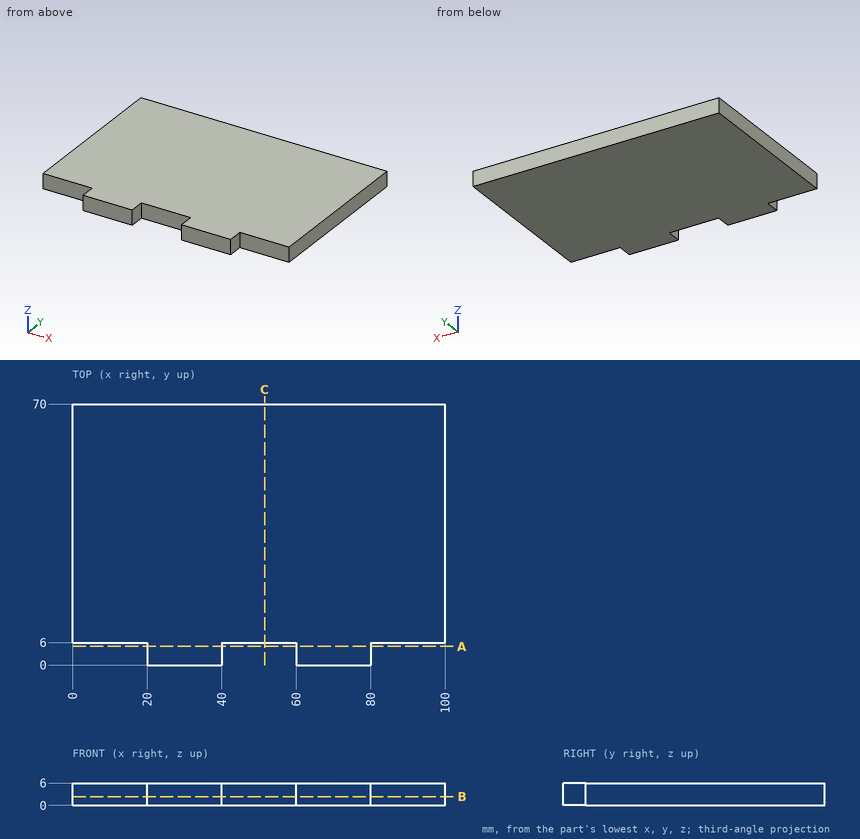
Input: dimensioned drawing with shaded views. Units: mm. Origin: part minimum x, y, z. Give positions to 0.01 mm unless a question says otherwise; leave off trailing zeros. Write each loop counter-clockwise with the first axis right and the second up, starting at its lowest first coordinate (ties: lowest second). Pieces come first, ordered by that corner, then holes. Notation, with made-up numbers: M 57.5,49.25 L 100.5,49.25 A20 ccw 100.5,57.25 Z; hole C 60.5,70 d9. An arc over 180 degrees is marked long. Return JSON: item names as keys, results as strings. Group by question number.
1) Material intervals for line 1 along Y through (x, z) = (15, 1.25), sorted ascending. Write a range as [from, to].
2) Pin query (flat end, axial travel): P1, Ø1.8, axis at y = 2.5, z = 2, coming from the +X side; P2, Ø2, axis at x = 69.5, y = 62, coming from the -Z side. Return the tip coordinate at first contact, or that it passes through.
3) Cut plane B-B, the plane z = 2.35. Output: boundary loops of the cut face in (x, y).
4) Cut plane C-C, the plane x = 51.5. Output: boundary loops of the cut face in (y, z), plus the area to 3 significant figures.
5) Cut plane A-A, the plane y = 5. Output: boundary loops of the cut face in (x, z).
Recorded:
{
 "1": {"line 1": "y = [6, 70]"},
 "2": {"P1": "stops at x = 80", "P2": "stops at z = 0"},
 "3": {"outline": "M 0,6 L 20,6 L 20,0 L 40,0 L 40,6 L 60,6 L 60,0 L 80,0 L 80,6 L 100,6 L 100,70 L 0,70 Z"},
 "4": {"outline": "M 6,0 L 70,0 L 70,6 L 6,6 Z", "area": "384 mm²"},
 "5": {"outline": "M 20,0 L 40,0 L 40,6 L 20,6 Z; M 60,0 L 80,0 L 80,6 L 60,6 Z"}
}
